Design review of the part shown in the three views and the two pictorial views. Dimensions are in mm from the part's minimum x, y and z. Round coordinates to 2 decimals unless told otherwise and drop trailing zeros. Loops run counter-clockwise (first coordinate to the right, second up) from the corner with the lowest first, then second, coordinate; pieces in that order, holes last. Notation, with made-up numbers: M 33.5,-5 L 86.5,-5 A19 cw 86.5,13 Z; hole C -10,34 d9. An arc over 180 degrees is marked long. Answer in a Markdown table with one row per item. Add a question column.
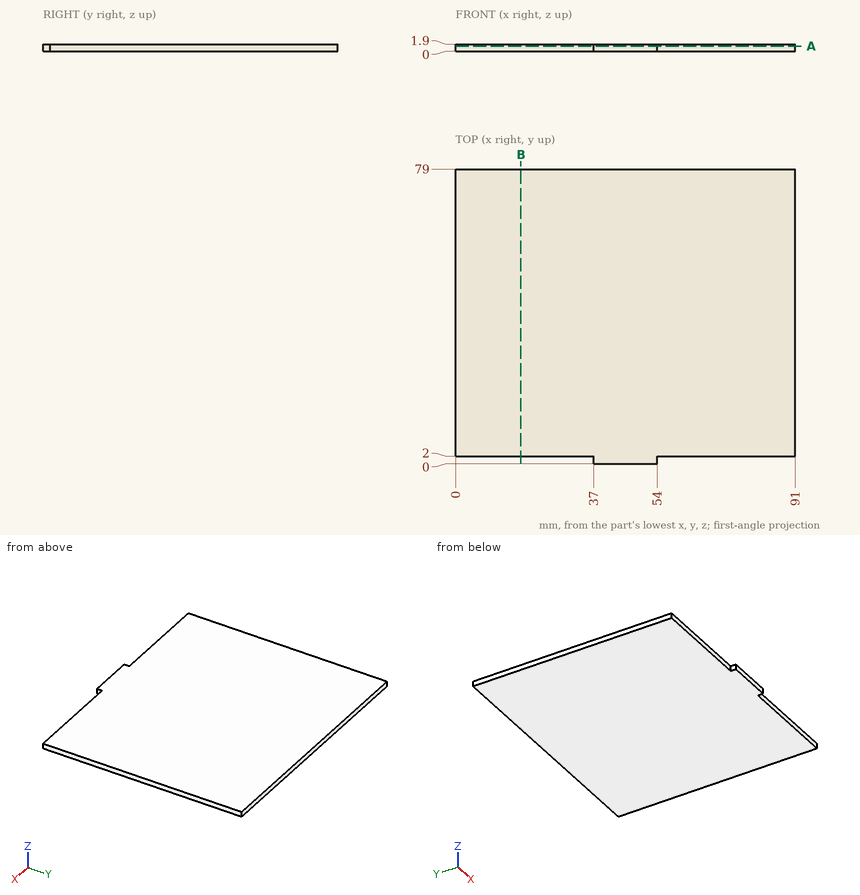
1. Take a section at B-B, the plane x = 17.5. State the section outline as (y, z) points, and give its area (3 significant figures).
2. To check wall thickness, follow probe 1 along Y at (x, z) = (35.5, 0.8). State the ranges of the line that lie inside material, in increasing order.
3. For pin 1 Ø1 at (x, z) = (23.5, 1) entering from -Y; pin 2 Ø8 at (x, y) = (69.5, 68) entering from -Z; pin 3 Ø0.6 at (y, z) = (0.5, 1) entering from -X; pin 4 Ø1 at (y, z) = (0.5, 1) entering from +X, all flat-tipped, find the tip position at first contact; note any pin that passes through.
4. Take a section at A-A, the plane z = 1.3. State the section outline as (x, y) points, and give its area (3 significant figures).
Check sheet entries:
| question | item | result |
|---|---|---|
| 1 | outline | M 2,0 L 79,0 L 79,1.9 L 2,1.9 Z |
| 1 | area | 146 mm^2 |
| 2 | probe 1 | y = 2 to 79 |
| 3 | pin 1 | stops at y = 2 |
| 3 | pin 2 | stops at z = 0 |
| 3 | pin 3 | stops at x = 37 |
| 3 | pin 4 | stops at x = 54 |
| 4 | outline | M 0,2 L 37,2 L 37,0 L 54,0 L 54,2 L 91,2 L 91,79 L 0,79 Z |
| 4 | area | 7,040 mm^2 |
